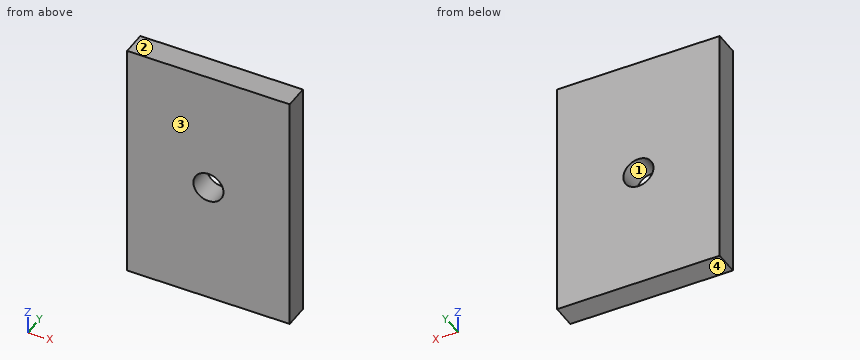
```python
from build123d import *

# Parameters (mm, degrees)
SKETCH_1_W          = 20
SKETCH_1_H          = 30
EXTRUDE_1_DEPTH     = 3
SKETCH_2_R          = 1.85
CUT_EXTRUDE_1_DEPTH = 3


with BuildPart() as part:
    # 草图1 → 凸台-拉伸1 (new body)
    with BuildSketch(Plane(origin=(0, 0, 0), x_dir=(1, 0, 0), z_dir=(0, 1, 0))):
        Rectangle(SKETCH_1_W, SKETCH_1_H)
    extrude(amount=EXTRUDE_1_DEPTH)

    # 草图2 → 切除-拉伸1 (cut)
    with BuildSketch(Plane(origin=(0, 3, 0), x_dir=(1, 0, 0), z_dir=(0, 1, 0))):
        with Locations(Location((0, 0, 0), (0, 0, 270))):
            Circle(SKETCH_2_R)
    extrude(amount=-CUT_EXTRUDE_1_DEPTH, mode=Mode.SUBTRACT)


solid = part.part
```
Build history of the part. All positions in model axes, mm. Face numbers are marked on the shaded views. Round coordinates to 2 decimals unless told otherwise and drop trailing zeros. Loops run counter-clockwise (first coordinate to the right, second up) from the corner with the lowest first, then second, coordinate; pieces in that order, holes last. Notation, with made-up numbers: M -6,-34 L 27,-34 A21 ccw 27,3 Z; hole C -4.5,-9 d8. An arc over 180 degrees is marked long. Answer as CSV lines item,"result".
1. Cut at A-A on x = 0. Write the cut outline in (y, z), then the cut area to 3 significant figures.
Resolved:
outline,"M 0,-15 L 3,-15 L 3,-1.85 L 0,-1.85 Z; M 0,1.85 L 3,1.85 L 3,15 L 0,15 Z"
area,"78.9 mm²"
2. Two-plate mould, pull along Z, no slides. Class the marked faces 1, 2, 3 and 4: released by +Z, released by -Z, zero draft, split by the parting line, or undercut.
Resolved:
face 1,"undercut"
face 2,"released by +Z"
face 3,"zero draft"
face 4,"released by -Z"
3. Wall check: probe 1 along X at (y, z) = (0.75, 0); probe 2 along Z at (x, y) = (0.25, 2.5). Give the ranges that are in metal, low to high. Write a range as [from, to].
Resolved:
probe 1,"x = [-10, -1.85], [1.85, 10]"
probe 2,"z = [-15, -1.83], [1.83, 15]"
4. Cut at B-B on z = 0. Write the cut outline in (x, y).
Resolved:
outline,"M -10,0 L -1.85,0 L -1.85,3 L -10,3 Z; M 1.85,0 L 10,0 L 10,3 L 1.85,3 Z"
5. Cut at C-C on y = 2.25. Write the cut outline in (x, z), then the cut area to 3 significant figures.
Resolved:
outline,"M -10,-15 L 10,-15 L 10,15 L -10,15 Z; hole C 0,0 d3.7"
area,"589 mm²"
